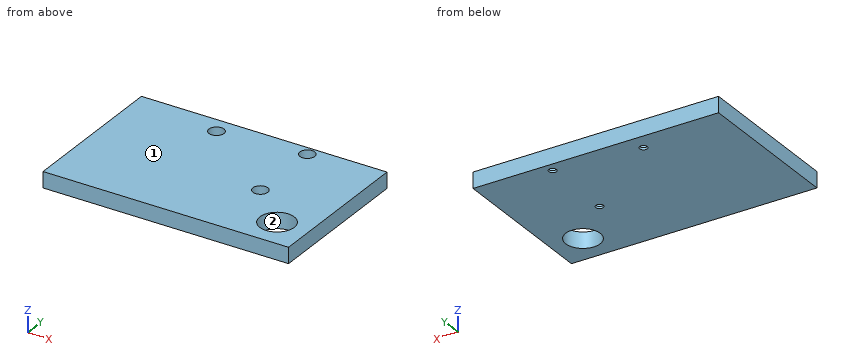
Autodesk Inventor part; units mm, degrees
ref_plane "Work Plane2" through (-44.4224, -5.9353, 6.9) normal (0, 0, -1) x (0, 1, 0)
ref_plane "YZ Plane" through (0, 0, 0) normal (1, 0, 0) x (0, 1, 0)
ref_plane "XZ Plane" through (0, 0, 0) normal (0, 1, 0) x (-1, 0, 0)
ref_plane "Work Plane1" through (0, 0, 0) normal (0, 0, 1) x (1, 0, 0)
sketch "Sketch1" plane through (0, 0, 0) normal (0, 0, 1) x (1, 0, 0)
  circle A0 centre (35.6776, 53.4286) radius 1.65 construction
  circle A1 centre (91.3776, 7.2647) radius 7.5 construction
  circle A2 centre (73.1776, 24.5117) radius 1.65 construction
  circle A3 centre (73.1776, 56.6946) radius 1.65 construction
  circle A4 centre (75.9087, -63.7578) radius 1.65 construction
  circle A5 centre (1.8224, -63.7578) radius 1.65 construction
  line L0 (105.1776, 60.9647) -> (-1.8224, 60.9647) construction
  line L1 (-1.8224, 60.9647) -> (-1.8224, -66.5509) construction
  line L2 (-1.8224, -66.5509) -> (78.1776, -66.5509) construction
  line L3 (78.1776, -66.5509) -> (78.1776, -30.5509) construction
  line L4 (78.1776, -30.5509) -> (105.1776, -30.5509) construction
  line L5 (105.1776, -30.5509) -> (105.1776, 60.9647) construction
  line L6 (105.1776, 60.9647) -> (-1.8224, 60.9647)
  line L7 (-1.8224, 60.9647) -> (-1.8224, -6.5353)
  line L8 (-1.8224, -6.5353) -> (105.1776, -6.5353)
  line L9 (105.1776, -6.5353) -> (105.1776, 60.9647)
  circle A6 centre (91.3776, 7.2647) radius 7.5
  circle A7 centre (73.1776, 56.6946) radius 1.65
  circle A8 centre (73.1776, 24.5117) radius 1.65
  circle A9 centre (35.6776, 53.4286) radius 1.65
  point P0 (0, 0)
  dimension "d0" = 13.8
ref_plane "Work Plane2" through (-44.4224, -5.9353, 6.9) normal (0, 0, -1) x (0, 1, 0)
extrude "Extrusion1" add sketch "Sketch1" along normal up to surface (6.9 mm away)
sketch "Sketch2" plane through (-1.8224, 60.9647, 6.9) normal (0, 0, 1) x (1, 0, 0)
  circle A0 centre (37.5, -7.536) radius 1.65
  circle A1 centre (75, -4.2701) radius 1.65
  circle A2 centre (75, -36.453) radius 1.65
  circle A3 centre (75, -4.2701) radius 3.25
  circle A4 centre (37.5, -7.536) radius 3.25
  circle A5 centre (75, -36.453) radius 3.25
  point P0 (1.8224, -60.9647)
  dimension "d3" = 6.5
  dimension "d4" = 6.5
  dimension "d5" = 6.5
extrude "Extrusion2" cut sketch "Sketch2" against normal blind 6
properties part number "10_MiniSPIM_Smarthponebase"
The model under review builds one solid part; all positions refer to its coordinate system, in mm. Face numbers are marked on the shaded views. Round coordinates to 2 decimals unless told otherwise and drop trailing zeros. Loops run counter-clockwise (first coordinate to the right, second up) from the corner with the lowest first, then second, coordinate; pieces in that order, holes last. Notation, with made-up numbers: (44, -22) -> (59, -22) arc R21 cw to (59, -7) -> close; hole circle Ø10 at (-25, 26). An arc over 180 degrees is marked (long way). Write item = value, one per line. Start each with the question number.
Item 1: Take a section at B-B on z = 4.5. Give the boundary of the cut face in (x, y).
Item 2: Take a section at C-C on y = 9. Give the boundary of the cut face in (x, z).
Item 3: To check wall thickness, follow L1, parallel to X at y = 56, z = 3.5; L2, parallel to Y at x = 89.5, z = 5.5; L3, parallel to X at y = 4.5, z = 6. State the ranges of each line that lie inside material, in increasing order.
Item 4: Take a section at A-A on x = 92.5. Give the boundary of the cut face in (y, z).
Item 5: Insertion check: pin 1 (3 mm diameter, centred on x = 73, y = 56, fed in from +Z). The pin has a flat end and moves straight along its axis. Give the tip position at first contact, or say it passes through.
Item 6: Mouldability with a two-part tool opening along X and no side actions: class the marked faces 1 and 2 as released by +X, released by -X, zero draft, split by the parting line, or undercut.
Result:
q1.outline = (-1.82, -6.54) -> (105.18, -6.54) -> (105.18, 60.96) -> (-1.82, 60.96) -> close; hole circle Ø6.5 at (35.68, 53.43); hole circle Ø6.5 at (73.18, 24.51); hole circle Ø6.5 at (73.18, 56.69); hole circle Ø15 at (91.38, 7.26)
q2.outline = (-1.82, 0) -> (84.08, 0) -> (84.08, 6.9) -> (-1.82, 6.9) -> close; (98.67, 0) -> (105.18, 0) -> (105.18, 6.9) -> (98.67, 6.9) -> close
q3.L1 = -1.82 to 33.69, 37.67 to 70, 76.35 to 105.18
q3.L2 = -6.54 to 0, 14.53 to 60.96
q3.L3 = -1.82 to 84.41, 98.35 to 105.18
q4.outline = (-6.54, 0) -> (-0.15, 0) -> (-0.15, 6.9) -> (-6.54, 6.9) -> close; (14.68, 0) -> (60.96, 0) -> (60.96, 6.9) -> (14.68, 6.9) -> close
q5.pin_1 = 0.9
q6.face_1 = zero draft
q6.face_2 = undercut
